Work out the finished part from the listing and answer in its coordinate system (mm). A direction names the side the tool comes from. Round coordinates to 2 decimals unless told otherwise and drop trailing zeros. Write each loop counter-clockwise with the first axis right and the second up, starting at its lowest first coordinate (ties: lowest second). Pieces come first, ordered by that corner, then holes. Notation, with made-up numbers: M -14,88 L 9,88 A26 cw 9,124 Z; hole C 76.25,59 d3. An arc over 180 degrees is marked long. Answer in a Markdown table with one row per item.
```python
from build123d import *

# Parameters (mm, degrees)
F0_W     = 34.925
F0_H     = 28.575
F1_DEPTH = 1.5875
F3_D     = 4.4958
F3_DEPTH = 12.7
F3_TIP   = 1.3506745855
F4_W     = 12.192
F4_H     = 28.575
F5_DEPTH = 3.175
F6_R     = 9.525
F7_DEPTH = 6.351


with BuildPart() as f1:
    # F0 (on Front) → F1 (new body, symmetric)
    with BuildSketch(Plane.XZ):
        Rectangle(F0_W, F0_H)
    extrude(amount=F1_DEPTH, both=True)

    # F3
    with Locations(Plane.XZ.offset(1.5875)):
        with Locations((-12.7, 9.525), (12.7, -9.525)):
            Hole(F3_D / 2, depth=F3_DEPTH)
            with Locations((0, 0, -(F3_DEPTH + F3_TIP / 2))):  # 118° drill point
                Cone(0, F3_D / 2, F3_TIP, mode=Mode.SUBTRACT)

    # F4 (on face) → F5 (join)
    with BuildSketch(Plane(origin=(0, 1.5875, 0), x_dir=(-1, 0, 0), z_dir=(0, 1, 0))):
        Rectangle(F4_W, F4_H)
    extrude(amount=F5_DEPTH)

    # F6 (on face) → F7 (cut, through all)
    with BuildSketch(Plane.XZ.offset(1.5875)):
        Circle(F6_R)
    extrude(amount=-F7_DEPTH, mode=Mode.SUBTRACT)


solid = f1.part
```
1. Determine the mould class of faces 1 (the flat face through (-6.096, 3, 11)), 2 (the flat face through (0, 1, -14.288)), 3 (the cylindrical face through (-10.454, 0.022, 9.624)) for opening direction Z: released by +Z, released by -Z, zero draft, split by the parting line, or undercut.
Calculated:
| item | result |
|---|---|
| face 1 | zero draft |
| face 2 | released by -Z |
| face 3 | undercut |
2. The part is cut by section C-C (y = 0.25). Count the separate pieces of the cut face and the enclosed holes in it, plus the area to 3 significant figures.
Calculated:
| item | result |
|---|---|
| separate pieces | 1 |
| enclosed holes | 3 |
| area | 681 mm² |
3. The part is cut by section B-B (x = 12.7). Determine the outline of the cut face in (y, z), plus the area to 3 significant figures.
Calculated:
| item | result |
|---|---|
| outline | M -1.59,-14.29 L 1.59,-14.29 L 1.59,-11.77 L -1.59,-11.77 Z; M -1.59,-7.28 L 1.59,-7.28 L 1.59,14.29 L -1.59,14.29 Z |
| area | 76.5 mm² |
4. Given pin 1 (2 mm diameter, centred on y = 2.5, z = -3.5, fed in from +X); pin 2 (1 mm diameter, centred on x = 4.5, z = 6.5, fed in from +Y); pin 3 (2.5 mm diameter, centred on y = 4, z = -10.5, fed in from +X); pin 4 (9 mm diameter, centred on x = -10, z = -3, fed in from +Y), each flat-ended and moving along its own axis, determine where each tip first touches the part or whether it passes through.
Calculated:
| item | result |
|---|---|
| pin 1 | stops at x = 17.46 |
| pin 2 | passes through |
| pin 3 | stops at x = 6.1 |
| pin 4 | stops at y = 1.59 |
5. A tool of negligible diameter and unlimited length cuts with its end or side. For faces 4 (the flat face through (0, 4.762, -12)), 5 (the flat face through (6.096, 3, 11)), 6 (the flat face through (-6.096, 3, -11)), from which of +Z, -Z, +X, -X, +Y, -Y can it reach the whole face along a straight path? Write none if from no direction.
Calculated:
| item | result |
|---|---|
| face 4 | +Z, -Z, +X, -X, +Y |
| face 5 | +Z, -Z, +X, +Y |
| face 6 | +Z, -Z, -X, +Y |
6. Consider line 1 along Z through (x, y) = (0, 2) (1 decimal); line 2 along Z through (x, y) = (12.5, -1); line 3 along X through (y, z) = (3.75, 8). Determine where each line is inside the solid, lowest interval first. Write a range as from..to.
Calculated:
| item | result |
|---|---|
| line 1 | z = -14.3..-9.5, 9.5..14.3 |
| line 2 | z = -14.29..-11.76, -7.29..14.29 |
| line 3 | x = -6.1..-5.17, 5.17..6.1 |
7. The part is cut by section D-D (z = -8.25). Determine the outline of the cut face in (x, y).
Calculated:
| item | result |
|---|---|
| outline | M -17.46,-1.59 L -4.76,-1.59 L -4.76,4.76 L -6.1,4.76 L -6.1,1.59 L -17.46,1.59 Z; M 4.76,-1.59 L 10.85,-1.59 L 10.85,1.59 L 6.1,1.59 L 6.1,4.76 L 4.76,4.76 Z; M 14.55,-1.59 L 17.46,-1.59 L 17.46,1.59 L 14.55,1.59 Z |
